from build123d import *

# Parameters (mm, degrees)
SKETCH_1_W          = 25.58
SKETCH_1_H          = 36
EXTRUDE_1_DEPTH     = 15
SKETCH_2_W          = 10
SKETCH_2_H          = 26
CUT_EXTRUDE_1_DEPTH = 35.689139511
HOLE_WIZARD_M2_1_D  = 2.4
FILLET_1_R          = 1
SKETCH_5_R          = 4.25
CUT_EXTRUDE_2_DEPTH = 1.5
HOLE_WIZARD_M2_2_D  = 2.4


with BuildPart() as part:
    # ｽｹｯﾁ1 → ﾎﾞｽ - 押し出し1 (new body)
    with BuildSketch(Plane.XY):
        Rectangle(SKETCH_1_W, SKETCH_1_H)
    extrude(amount=EXTRUDE_1_DEPTH)

    # ｽｹｯﾁ2 → ｶｯﾄ - 押し出し1 (cut, through all)
    with BuildSketch(Plane.ZY.offset(12.79)):
        with Locations((10, 0)):
            Rectangle(SKETCH_2_W, SKETCH_2_H)
    extrude(amount=-CUT_EXTRUDE_1_DEPTH, mode=Mode.SUBTRACT)

    # M2 すきま穴1 (through all)
    with Locations(Plane(origin=(0, 18, 0), x_dir=(1, 0, 0), z_dir=(0, 1, 0))):
        with Locations((-10.5, -12), (10.5, -12)):
            Hole(HOLE_WIZARD_M2_1_D / 2)

    # ﾌｨﾚｯﾄ1
    fillet_1_edges = [part.edges().sort_by_distance(p)[0] for p in [
        (-12.79, 0, 0),
        (12.79, 0, 0),
    ]]
    fillet(fillet_1_edges, radius=FILLET_1_R)

    # ｽｹｯﾁ5 → ｶｯﾄ - 押し出し2 (cut)
    with BuildSketch(Plane(origin=(0, 0, 0), x_dir=(-1, 0, 0), z_dir=(0, 0, -1))):
        Circle(SKETCH_5_R)
    extrude(amount=-CUT_EXTRUDE_2_DEPTH, mode=Mode.SUBTRACT)

    # M2 すきま穴2 (through all)
    with Locations(Plane.XY.offset(5)):
        with Locations((4.242640687, 4.242640687), (-4.242640687, -4.242640687), (4.242640687, -4.242640687), (-4.242640687, 4.242640687)):
            Hole(HOLE_WIZARD_M2_2_D / 2)


solid = part.part
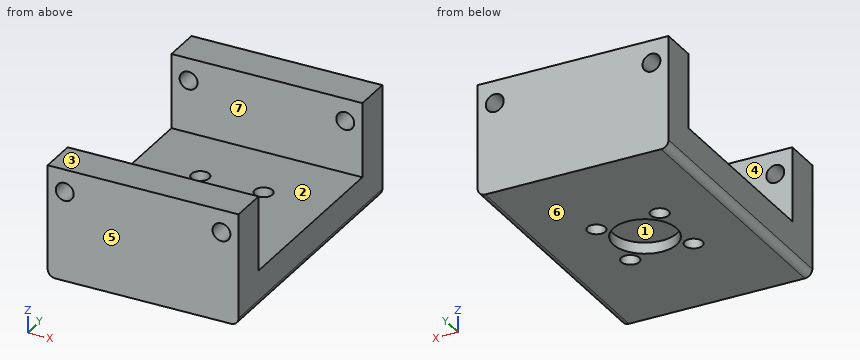
Input: part model. Units: mm. Frame: model coordinates. Face numbers are marked on the shaded views. A direction names the side the tool comes from. Coordinates: 2 decimals unless noted, no trailing zeros. Order: outer loops, then holes, each group sorted by start corner. A loop starts at its lowest first (then second) coordinate and runs counter-clockwise, first axis right, second up. Notation, with made-up numbers: M 53.5,-21 L 64.5,-21 A23 cw 64.5,14 Z; hole C 26.5,-7.5 d10. An arc over 180 degrees is marked long. Answer in a Markdown table with one row per item.
(1) Draft query along Y for the marked faces 4, 5, 6 and 7. Return one class per face: pulls with the +Y half, pulls with the -Y half, needs draft (parallel to the pull), parting line crosses it, or undercut.
Numbers:
| item | result |
|---|---|
| face 4 | undercut |
| face 5 | pulls with the -Y half |
| face 6 | needs draft |
| face 7 | undercut |
(2) Section query A-A, the plane z = 7. Output: boundary loops of the cut face in (x, y), plus the area to 3 significant figures.
Numbers:
| item | result |
|---|---|
| outline | M -12.79,-18 L 12.79,-18 L 12.79,-13 L -12.79,-13 Z; M -12.79,13 L 12.79,13 L 12.79,18 L -12.79,18 Z |
| area | 256 mm^2 |
(3) Contact query for flat-ended pins moving along their axis: pin 1 Ø3 at (x, z) = (-10.5, 12) entering from -Y; pin 2 Ø2 at (x, y) = (4.24, -4.24) entering from -Z; pin 3 Ø7.5 at (x, y) = (2.5, -0.5) entering from +Z; pin 4 Ø2.5 at (x, y) = (-1.5, 0) entering from -Z. Output: stop coordinate, or through.
Numbers:
| item | result |
|---|---|
| pin 1 | stops at y = -18 |
| pin 2 | passes through |
| pin 3 | stops at z = 5 |
| pin 4 | stops at z = 1.5 |
(4) Section query C-C, the plane z = 12. Output: boundary loops of the cut face in (x, y), plus the area to 3 significant figures.
Numbers:
| item | result |
|---|---|
| outline | M -12.79,-18 L -11.7,-18 L -11.7,-13 L -12.79,-13 Z; M -12.79,13 L -11.7,13 L -11.7,18 L -12.79,18 Z; M -9.3,-18 L 9.3,-18 L 9.3,-13 L -9.3,-13 Z; M -9.3,13 L 9.3,13 L 9.3,18 L -9.3,18 Z; M 11.7,-18 L 12.79,-18 L 12.79,-13 L 11.7,-13 Z; M 11.7,13 L 12.79,13 L 12.79,18 L 11.7,18 Z |
| area | 208 mm^2 |
(5) Material intervals for line 1 (Z direction, x = 10.5, y = -16.9); line 2 (X direction, y = 4.5, z = 2.5); line 3 (Y direction, x = 1, z = 6.75), sorted ascending. Write a range as [from, to].
Numbers:
| item | result |
|---|---|
| line 1 | z = [0, 10.8], [13.2, 15] |
| line 2 | x = [-12.79, -5.41], [-3.07, 3.07], [5.41, 12.79] |
| line 3 | y = [-18, -13], [13, 18] |
(6) Access query for the marked faces 1, 2 and 3. Directions: +Z, -Z, +X, -X, +Y, -Y. A direction counts if a zero-diameter tool reaches every point of the face in a straight line with its end or side. Return the directions, or none.
Numbers:
| item | result |
|---|---|
| face 1 | -Z |
| face 2 | +Z, +X, -X |
| face 3 | +Z, +X, -X, +Y, -Y |
(7) Section query B-B, the plane x = 10.5. Output: boundary loops of the cut face in (y, z).
Numbers:
| item | result |
|---|---|
| outline | M -18,0 L 18,0 L 18,10.8 L 13,10.8 L 13,5 L -13,5 L -13,10.8 L -18,10.8 Z; M -18,13.2 L -13,13.2 L -13,15 L -18,15 Z; M 13,13.2 L 18,13.2 L 18,15 L 13,15 Z |
(8) Section query D-D, the plane y = 0. Output: boundary loops of the cut face in (x, z), plus the area to 3 significant figures.
Numbers:
| item | result |
|---|---|
| outline | M -12.79,1 A1 ccw -11.79,0 L -4.25,0 L -4.25,1.5 L 4.25,1.5 L 4.25,0 L 11.79,0 A1 ccw 12.79,1 L 12.79,5 L -12.79,5 Z |
| area | 115 mm^2 |
